Verification items for the finished model (mm, model axes). Round coordinates to 2 decimals unless told otherwise and drop trailing zeros. Write each loop counter-clockwise with the first axis right and the second up, starting at its lowest first coordinate (ties: lowest second). Pieces come first, ordered by that corner, then holes. Notation, with made-up numbers: M -6,35.5 L 40,35.5 A12 ccw 40,45.5 Z; hole C 54,6 d5. An arc over 180 degrees is marked long. One line per item, written item: value. Start each with the question number.
Item 1: Section check C-C, the plane y = -6.5. Record the cut outline in (x, z), then the cut area to 3 significant figures.
Item 2: Thickness scan on probe 1 along Z at (x, y) = (0, -6.5); probe 2 along X at (y, z) = (-2.75, 60); probe 3 along Z at (x, y) = (-9, -8.5). Record the ranges inside material, lowest first. Write a range as from..to.
Item 3: Section check D-D, the plane z = 86. Record the cut outline in (x, y).
Item 4: Section check B-B, the plane z = 60. Record the cut outline in (x, y), then the cut area to 3 significant figures.
Item 5: Section check A-A, the plane x = -12. Record the cut outline in (y, z).
Item 6: Gauge pin test, flat end, axial feed: pin 1 (1 mm diameter, centred on x = 7, z = 78.5, fed in from +Y). Record the tip position at first contact, or that the pin passes through.
from build123d import *

# Parameters (mm, degrees)
F0_W          = 70
F0_H          = 200
F1_DEPTH      = 10
F2_R          = 15
F3_DEPTH      = 218
F3_DEPTH_BACK = 25
F4_R          = 20


# Not quite as in the source:
# - an extrude ends at something that could not be found from the text; its depth is read off the source's solid


with BuildPart() as f1:
    # F0 (on Front) → F1 (new body)
    with BuildSketch(Plane.XZ):
        Rectangle(F0_W, F0_H)
    extrude(amount=F1_DEPTH)

    # F2 (on Front) → F3 (cut, two sides)
    with BuildSketch(Plane.XZ) as f3_sk:
        with Locations((0, 60)):
            Circle(F2_R)
    extrude(amount=-F3_DEPTH, mode=Mode.SUBTRACT)
    extrude(f3_sk.sketch, amount=F3_DEPTH_BACK, mode=Mode.SUBTRACT)

    # F4
    f4_edges = [f1.edges().sort_by_distance(p)[0] for p in [
        (-35, -5, 100),
        (35, -5, 100),
    ]]
    fillet(f4_edges, radius=F4_R)


solid = f1.part
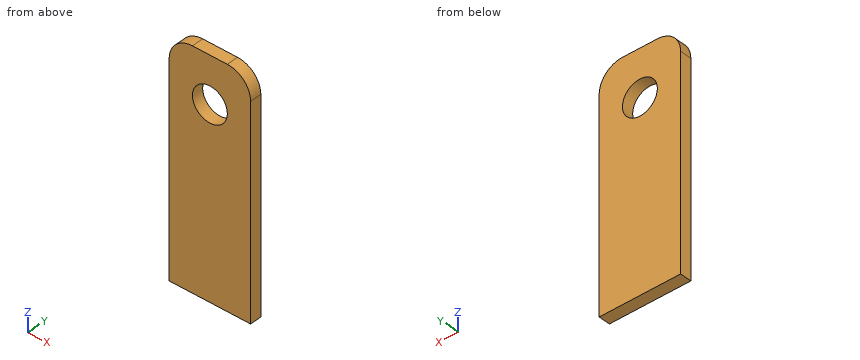
Response values:
1. outline: M -35,-100 L 35,-100 L 35,80 A20 ccw 15,100 L -15,100 A20 ccw -35,80 Z; hole C 0,60 d30
1. area: 13,100 mm2
2. probe 1: z = -100..45, 75..100
2. probe 2: x = -35..-15, 15..35
2. probe 3: z = -100..48, 72..100
3. outline: M -34.08,-10 L 34.08,-10 L 34.08,0 L -34.08,0 Z
4. outline: M -35,-10 L -15,-10 L -15,0 L -35,0 Z; M 15,-10 L 35,-10 L 35,0 L 15,0 Z
4. area: 400 mm2
5. outline: M -10,-100 L 0,-100 L 0,51 L -10,51 Z; M -10,69 L 0,69 L 0,100 L -10,100 Z
6. pin 1: stops at y = 0
